Verification items for this drawing (mm, ordinates from the low corner). Round coordinates to 2 decimals unless told otherwise and drop trailing zeros. Order: outer loops, then holes, each group sorted by start corner. A loop starts at its lowest first (then second) coordinate and runs counter-clockwise, first axis right, second up. Notation, with made-up numbers: (82, 27.25) - (116, 27.25) arc R18 cw to (116, 42.25) - close; hole circle Ø6 at (-3, 31). An arc over 180 degrees is marked (long way). Use a Markdown table: item, result. Add a question column.
(1) Gauge pin test, flat end, axial feed: P1, Ø2, axis at y = 61, z = 7, coming from the -X side (1 decimal). Record the tip position at first contact, or that the pin passes through.
(2) Thickness scan on line 1 along Y through (x, z) = (431.8, 3.5); line 2 along X through (y, z) = (24.5, 1.25) (1 decimal); line 3 along X through (y, z) = (31, 4) (1 decimal). Record the ranges inside material, lowest first. Write a range as [from, to].
(3) Section check C-C on y = 9.5. Record the boundary of the cut face in (x, z), then the cut area to 3 significant figures.
(4) Section check B-B on z = 5. Give the number of separate pieces and of enclosed holes in the cut face, then the cut area to 3 significant figures.
(5) Section check A-A on x = 431.8. Record the boundary of the cut face in (y, z).
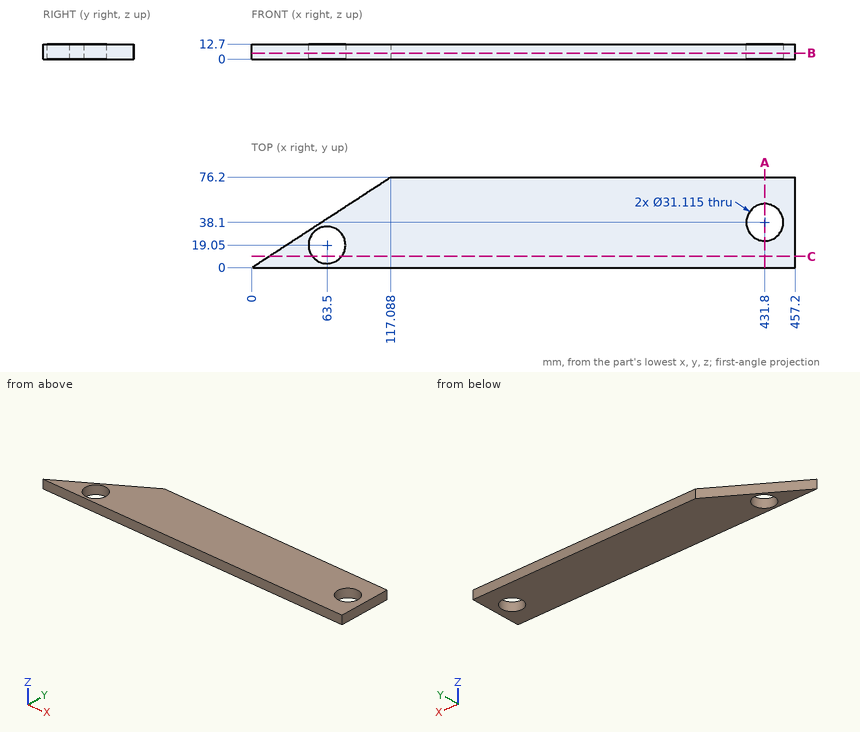
Check sheet entries:
| question | item | result |
|---|---|---|
| 1 | P1 | stops at x = 92.2 |
| 2 | line 1 | y = [0, 22.54], [53.66, 76.2] |
| 2 | line 2 | x = [37.6, 48.9], [78.1, 424.2], [439.4, 457.2] |
| 2 | line 3 | x = [47.6, 53.5], [73.5, 418], [445.6, 457.2] |
| 3 | outline | (14.6, 0) - (51.22, 0) - (51.22, 12.7) - (14.6, 12.7) - close; (75.78, 0) - (457.2, 0) - (457.2, 12.7) - (75.78, 12.7) - close |
| 3 | area | 5,310 mm2 |
| 4 | separate pieces | 1 |
| 4 | enclosed holes | 2 |
| 4 | area | 28,900 mm2 |
| 5 | outline | (0, 0) - (22.54, 0) - (22.54, 12.7) - (0, 12.7) - close; (53.66, 0) - (76.2, 0) - (76.2, 12.7) - (53.66, 12.7) - close |
